Can you work these out from the model? Positions are in its coordinate system, mm. A direction names the side the tool comes from. Coordinates: 2 decimals unless noted, no trailing zeros. Order: outer loops, then holes, each group sorted by start corner. A loop starts at its lowest first (then second) coordinate and runs counter-clockwise, first axis right, second up. Notation, with made-up numbers: (54, 50) -> (88, 50) arc R17 cw to (88, 62) -> close; hole circle Ø8 at (10, 10.25). An arc over 180 degrees is marked (long way). Answer in a Markdown table with one row per item. Add a question column.
1. We'd pull the mould along Z, two halves only. Please class faces 1 (the face through (13.577, 1.232, 8.626)), 2 (the face through (35, 1, 0)), 3 (the face through (28.041, 1.232, 9.797)), 4 (the face through (24.4, 1.23, -2.13)): pulls with the +Z half, pulls with the -Z half, needs draft (parallel to the pull), parting line crosses it, or undercut.
2. Imagine slicing it at A-A on x = 31.5. Write out the boundary of the cut face in (y, z).
3. If I drill on line 1 along Y through (x, z) = (-18, -5); line 2 along X through (y, z) = (0.5, -0.25); line 3 along X through (y, z) = (1.25, 3.5), over which ranges is the centre line in solid material (lowest first)? Write a range as [from, to].
4. Will these pins go through, and if not, where does the flat tip stop? pin 1 (2 mm diameter, centred on x = 33, y = 2, fed in from -Z); pin 2 (2 mm diameter, centred on x = -10.5, y = 1.5, fed in from +Z); pin 3 (1.1 mm diameter, centred on y = 1.5, z = -0.5, fed in from -X); pin 4 (8.5 mm diameter, centred on x = -10, z = -2.5, fed in from +Y).
5. Imagine slicing it at C-C on x = -24. Write out the boundary of the cut face in (y, z), plus the area to 3 significant figures.
6. On a 3-axis mill with a long thin cutter (end or side, diameter ignored), from which of +Z, -Z, +X, -X, +Y, -Y can I reach the whole of each face in a straight line? I mean faces 5 (the face through (8.601, 1.232, 12.115)), 6 (the face through (8.347, 1.232, -7.078)), 7 (the face through (32, 1, 9.7)), 8 (the face through (21, 0.5, 11)). Say none if no direction works.
7. Imagine slicing it at B-B on y = 1.8. State how many separate pieces and enclosed holes the cut face has, plus the area to 3 significant figures.
from build123d import *

# Parameters (mm, degrees)
SKETCH1_R           = 1.3
SKETCH1_R_2         = 1
SKETCH1_R_3         = 4.5
BOSS_EXTRUDE1_DEPTH = 2.5
SKETCH3_R           = 6
SKETCH3_R_2         = 3.75
BOSS_EXTRUDE2_DEPTH = 2
SKETCH4_R           = 4.5
SKETCH4_R_2         = 3.75
CUT_EXTRUDE1_DEPTH  = 1
CHAMFER1_SIZE       = 0.5
SKETCH6_R           = 3
CUT_EXTRUDE2_DEPTH  = 0.5


with BuildPart() as part:
    # Sketch1 → Boss-Extrude1 (new body)
    with BuildSketch(Plane(origin=(0, 0, 0), x_dir=(1, 0, 0), z_dir=(0, 1, 0))):
        with BuildLine():
            Line((35, 9.7), (35, -9.7))
            Line((35, -9.7), (28.656580513, -9.7))
            ThreePointArc((28.656580513, -9.7), (28.032756183, -9.799778117), (27.471175871, -10.089156794))
            Line((27.471175871, -10.089156794), (22.667160445, -13.62438739))
            ThreePointArc((22.667160445, -13.62438739), (20.936486005, -14.401466515), (19.039367435, -14.396259626))
            Line((19.039367435, -14.396259626), (-2.134739034, -9.769487666))
            ThreePointArc((-2.134739034, -9.769487666), (-2.213274492, -9.751995489), (-2.291666667, -9.733871989))
            Line((-2.291666667, -9.733871989), (-25.03125, -4.380242395))
            ThreePointArc((-25.03125, -4.380242395), (-28.5, 0), (-25.03125, 4.380242395))
            Line((-25.03125, 4.380242395), (-2.291666667, 9.733871989))
            ThreePointArc((-2.291666667, 9.733871989), (-2.213276651, 9.751994999), (-2.13474336, 9.769486721))
            Line((-2.13474336, 9.769486721), (19.039365488, 14.396269024))
            ThreePointArc((19.039365488, 14.396269024), (20.936487661, 14.401475987), (22.667164776, 13.624394026))
            Line((22.667164776, 13.624394026), (27.47117527, 10.089158211))
            ThreePointArc((27.47117527, 10.089158211), (28.032756372, 9.799778489), (28.656581837, 9.7))
            Line((28.656581837, 9.7), (35, 9.7))
        make_face()
        with Locations(Location((31.5, 6.7, 0), (0, 0, 270))):
            Circle(SKETCH1_R, mode=Mode.SUBTRACT)
        with Locations(Location((31.5, -6.7, 0), (0, 0, 270))):
            Circle(SKETCH1_R, mode=Mode.SUBTRACT)
        with Locations(Location((20, 10, 0), (0, 0, 270))):
            Circle(SKETCH1_R, mode=Mode.SUBTRACT)
        with Locations(Location((20, -9.999990176, 0), (0, 0, 270))):
            Circle(SKETCH1_R_2, mode=Mode.SUBTRACT)
        with Locations(Location((0, 0, 0), (0, 0, 270))):
            Circle(SKETCH1_R_3, mode=Mode.SUBTRACT)
        with Locations(Location((-24, 0, 0), (0, 0, 270))):
            Circle(SKETCH1_R, mode=Mode.SUBTRACT)
        with Locations(Location((22.5, -6.7, 0), (0, 0, 270))):
            Circle(SKETCH1_R_2, mode=Mode.SUBTRACT)
        with BuildLine():
            Line((9.772066478, 8.276878442), (12.216286037, 8.810968065))
            ThreePointArc((12.216286037, 8.810968065), (13.559618748, 8.634777191), (14.482426032, 7.642803041))
            ThreePointArc((14.482426032, 7.642803041), (16.274630398, 5.296637232), (18.968838896, 4.089271891))
            ThreePointArc((18.968838896, 4.089271891), (19.472295347, 3.930738723), (19.916745685, 3.646019459))
            ThreePointArc((19.916745685, 3.646019459), (21.124485944, 2.943943413), (22.5, 2.7))
            Line((22.5, 2.7), (23, 2.7))
            ThreePointArc((23, 2.7), (24.414213562, 2.114213562), (25, 0.7))
            Line((25, 0.7), (25, -0.7))
            ThreePointArc((25, -0.7), (24.414213562, -2.114213562), (23, -2.7))
            Line((23, -2.7), (22.5, -2.7))
            ThreePointArc((22.5, -2.7), (21.124485854, -2.943943446), (19.916745538, -3.646019583))
            ThreePointArc((19.916745538, -3.646019583), (19.472295389, -3.930738787), (18.968839153, -4.089271995))
            ThreePointArc((18.968839153, -4.089271995), (16.274635438, -5.296635948), (14.482434575, -7.642798226))
            ThreePointArc((14.482434575, -7.642798226), (13.559627706, -8.634772461), (12.216295281, -8.810963823))
            Line((12.216295281, -8.810963823), (9.772070143, -8.276874115))
            ThreePointArc((9.772070143, -8.276874115), (8.357168863, -7.102458424), (8.499181625, -5.269147152))
            ThreePointArc((8.499181625, -5.269147152), (10, 2.214e-06), (8.499179292, 5.269150915))
            ThreePointArc((8.499179292, 5.269150915), (8.357165718, 7.102462125), (9.772066478, 8.276878442))
        make_face(mode=Mode.SUBTRACT)
        with BuildLine():
            Line((-17.912878788, -1.946774398), (-12.387619024, -3.247598329))
            ThreePointArc((-12.387619024, -3.247598329), (-10.604369925, -2.799022253), (-9.941071409, -1.084019943))
            ThreePointArc((-9.941071409, -1.084019943), (-10, 0), (-9.941071409, 1.084019943))
            ThreePointArc((-9.941071409, 1.084019943), (-10.604369925, 2.799022253), (-12.387619024, 3.247598329))
            Line((-12.387619024, 3.247598329), (-17.912878788, 1.946774398))
            ThreePointArc((-17.912878788, 1.946774398), (-19.454545455, 0), (-17.912878788, -1.946774398))
        make_face(mode=Mode.SUBTRACT)
    extrude(amount=BOSS_EXTRUDE1_DEPTH)

    # Sketch3 → Boss-Extrude2 (add)
    with BuildSketch(Plane(origin=(0, 2.5, 0), x_dir=(1, 0, 0), z_dir=(0, 1, 0))):
        with Locations(Location((0, 0, 0), (0, 0, 90))):
            Circle(SKETCH3_R)
        with Locations(Location((0, 0, 0), (0, 0, 270))):
            Circle(SKETCH3_R_2, mode=Mode.SUBTRACT)
    extrude(amount=BOSS_EXTRUDE2_DEPTH)

    # Sketch4 → Cut-Extrude1 (cut)
    with BuildSketch(Plane.XZ.offset(-2.5)):
        with Locations(Location((0, 0, 0), (0, 0, 270))):
            Circle(SKETCH4_R)
        with Locations(Location((0, 0, 0), (0, 0, 270))):
            Circle(SKETCH4_R_2, mode=Mode.SUBTRACT)
    extrude(amount=-CUT_EXTRUDE1_DEPTH, mode=Mode.SUBTRACT)

    # Chamfer1
    chamfer1_edges = [part.edges().sort_by_distance(p)[0] for p in [
        (0, 4.5, 6),
    ]]
    chamfer(chamfer1_edges, length=CHAMFER1_SIZE)

    # Sketch6 → Cut-Extrude2 (cut)
    with BuildSketch(Plane.XZ):
        with Locations(Location((20, 9.999990176, 0), (0, 0, 270))):
            Circle(SKETCH6_R)
        with Locations(Location((20, -10, 0), (0, 0, 270))):
            Circle(SKETCH6_R)
    extrude(amount=-CUT_EXTRUDE2_DEPTH, mode=Mode.SUBTRACT)


solid = part.part
Answers follow:
| question | item | result |
|---|---|---|
| 1 | face 1 | undercut |
| 1 | face 2 | needs draft |
| 1 | face 3 | pulls with the +Z half |
| 1 | face 4 | undercut |
| 2 | outline | (0, -9.7) -> (2.5, -9.7) -> (2.5, -8) -> (0, -8) -> close; (0, -5.4) -> (2.5, -5.4) -> (2.5, 5.4) -> (0, 5.4) -> close; (0, 8) -> (2.5, 8) -> (2.5, 9.7) -> (0, 9.7) -> close |
| 3 | line 1 | y = [0, 2.5] |
| 3 | line 2 | x = [-28.49, -25.28], [-22.72, -19.44], [-10, -4.49], [4.49, 10], [25, 35] |
| 3 | line 3 | x = [-26.83, -2.83], [2.83, 9.37], [20.1, 35] |
| 4 | pin 1 | stops at z = -9.7 |
| 4 | pin 2 | stops at z = 8.04 |
| 4 | pin 3 | stops at x = -28.5 |
| 4 | pin 4 | stops at y = 2.5 |
| 5 | outline | (0, -4.62) -> (2.5, -4.62) -> (2.5, -1.3) -> (0, -1.3) -> close; (0, 1.3) -> (2.5, 1.3) -> (2.5, 4.62) -> (0, 4.62) -> close |
| 5 | area | 16.6 mm² |
| 6 | face 5 | +Z, -X, +Y, -Y |
| 6 | face 6 | +Y, -Y |
| 6 | face 7 | +Z, +X, +Y, -Y |
| 6 | face 8 | -Y |
| 7 | separate pieces | 1 |
| 7 | enclosed holes | 9 |
| 7 | area | 911 mm² |
